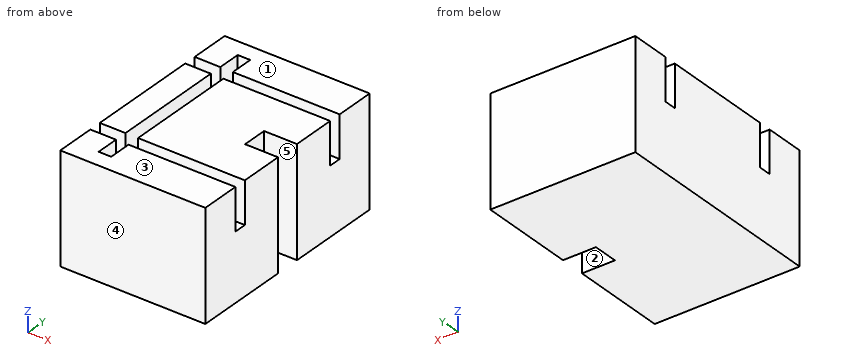
```python
from build123d import *

# Parameters (mm, degrees)
BOSS_EXTRUDE1_DEPTH = 13
SKETCH2_W           = 12.743753884
SKETCH2_H           = 1.5
SKETCH2_W_2         = 1.5
SKETCH2_H_2         = 2.75
SKETCH2_W_3         = 3.0625
SKETCH2_H_3         = 13.5
CUT_EXTRUDE1_DEPTH  = 5


with BuildPart() as part:
    # Sketch1 → Boss-Extrude1 (new body)
    with BuildSketch(Plane.XY):
        Polygon((10.243753884, 1.5), (10.243753884, 13), (8.5625, 13), (7.0625, 13), (-7.0625, 13), (-7.0625, -13), (7.0625, -13), (8.5625, -13), (10.243753884, -13), (10.243753884, -1.5), (9.3125, -1.5), (6.3125, -1.5), (6.3125, 1.5), (9.3125, 1.5), align=None)
    extrude(amount=BOSS_EXTRUDE1_DEPTH)

    # Sketch2 → Cut-Extrude1 (cut)
    with BuildSketch(Plane.XY.offset(13)):
        with Locations((3.871876942, 7.5)):
            Rectangle(SKETCH2_W, SKETCH2_H)
        with Locations((-3.25, 9.625)):
            Rectangle(SKETCH2_W_2, SKETCH2_H_2)
        with Locations((-5.53125, 7.5)):
            Rectangle(SKETCH2_W_3, SKETCH2_H)
        with Locations((-3.25, 7.5)):
            Rectangle(SKETCH2_W_2, SKETCH2_H)
        with Locations((-3.25, 0)):
            Rectangle(SKETCH2_W_2, SKETCH2_H_3)
        with Locations((-3.25, -9.625)):
            Rectangle(SKETCH2_W_2, SKETCH2_H_2)
        with Locations((-3.25, -7.5)):
            Rectangle(SKETCH2_W_2, SKETCH2_H)
        with Locations((-5.53125, -7.5)):
            Rectangle(SKETCH2_W_3, SKETCH2_H)
        with Locations((3.871876942, -7.5)):
            Rectangle(SKETCH2_W, SKETCH2_H)
    extrude(amount=-CUT_EXTRUDE1_DEPTH, mode=Mode.SUBTRACT)


solid = part.part
```
Build history of the part. All positions in model axes, mm. Face numbers are marked on the shaded views. A direction names the side the tool comes from. Give positions to 0.01 mm unless a question says otherwise; leave off trailing zeros. Loops run counter-clockwise (first coordinate to the right, second up) from the corner with the lowest first, then second, coordinate; pieces in that order, holes last.
1) Band-saw the part on A-A on x = 8.75. List the corners of the cut face in (y, z).
Values follow:
outline: (-13, 0) - (-1.5, 0) - (-1.5, 13) - (-6.75, 13) - (-6.75, 8) - (-8.25, 8) - (-8.25, 13) - (-13, 13) - close; (1.5, 0) - (13, 0) - (13, 13) - (8.25, 13) - (8.25, 8) - (6.75, 8) - (6.75, 13) - (1.5, 13) - close
2) Band-saw the part on D-D on x = 1.5. List the corners of the cut face in (y, z).
Values follow:
outline: (-13, 0) - (13, 0) - (13, 13) - (8.25, 13) - (8.25, 8) - (6.75, 8) - (6.75, 13) - (-6.75, 13) - (-6.75, 8) - (-8.25, 8) - (-8.25, 13) - (-13, 13) - close
3) 3-axis set-ups, long thin cutter, end or side, ignore diameter. For the marked faces 1 and 2: which of +Z, -Z, +X, -X, +Y, -Y reach the whole face in a straight line?
Values follow:
face 1: +Z, +X, -X, +Y, -Y
face 2: +Z, -Z, +X
4) Probe line 1 along Y through (x, z) = (3.5, 8.5); line 2 along Y through (x, z) = (6.75, 8.25); line 3 along X through (y, z) = (2.75, 8.25). List the from-to ranges inside material, lowest first.
Values follow:
line 1: y = -13 to -8.25, -6.75 to 6.75, 8.25 to 13
line 2: y = -13 to -8.25, -6.75 to -1.5, 1.5 to 6.75, 8.25 to 13
line 3: x = -7.06 to -4, -2.5 to 10.24
5) Band-saw the part on B-B on z = 9.25. List the corners of the cut face in (x, y), then the cut area to 3 significant figures.
Values follow:
outline: (-7.06, -13) - (10.24, -13) - (10.24, -8.25) - (-2.5, -8.25) - (-2.5, -11) - (-4, -11) - (-4, -8.25) - (-7.06, -8.25) - close; (-7.06, -6.75) - (-4, -6.75) - (-4, 6.75) - (-7.06, 6.75) - close; (-7.06, 8.25) - (-4, 8.25) - (-4, 11) - (-2.5, 11) - (-2.5, 8.25) - (10.24, 8.25) - (10.24, 13) - (-7.06, 13) - close; (-2.5, -6.75) - (10.24, -6.75) - (10.24, -1.5) - (6.31, -1.5) - (6.31, 1.5) - (10.24, 1.5) - (10.24, 6.75) - (-2.5, 6.75) - close
area: 358 mm2
6) Two-plate mould, pull along Y, no slides. Class the marked faces 3, 4 and 5: released by +Y, released by -Y, zero draft, split by the parting line, or undercut.
Values follow:
face 3: zero draft
face 4: released by -Y
face 5: undercut
7) Band-saw the part on C-C on y = -0.25. List the corners of the cut face in (x, z), then the cut area to 3 significant figures.
Values follow:
outline: (-7.06, 0) - (6.31, 0) - (6.31, 13) - (-2.5, 13) - (-2.5, 8) - (-4, 8) - (-4, 13) - (-7.06, 13) - close
area: 166 mm2
8) Drop a flat-ended pin along its axis: P1, Ø1.5, axis at x = -4.5, y = -7.5, coming from the -Z side. Give the stop position or say it passes through.
Values follow:
P1: stops at z = 0
